from build123d import *

# Parameters (mm, degrees)
F0_R     = 1.475
F1_DEPTH = 10
F3_DEPTH = 3


with BuildPart() as f1:
    # F0 (on Front) → F1 (new body)
    with BuildSketch(Plane.XZ):
        Circle(F0_R)
    extrude(amount=F1_DEPTH)

    # F2 (on face) → F3 (cut)
    with BuildSketch(Plane(origin=(0, 0, 0), x_dir=(-1, 0, 0), z_dir=(0, 1, 0))):
        Polygon((-1.073836, 0.037674), (-0.569545, -0.911132), (0.504291, -0.948806), (1.073836, -0.037674), (0.569545, 0.911132), (-0.504291, 0.948806), align=None)
    extrude(amount=-F3_DEPTH, mode=Mode.SUBTRACT)


solid = f1.part
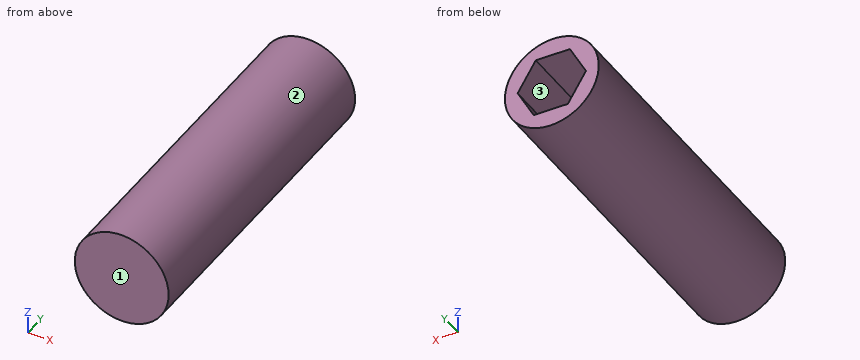
Can you work these out from the model? Positions are in its coordinate system, mm. Face numbers are marked on the shaded views. Give positions to 0.01 mm unless a question says otherwise; leave off trailing zeros. Loops run counter-clockwise (first coordinate to the right, second up) from the corner with the lowest first, then second, coordinate; pieces in that order, holes last. Notation, with made-up numbers: (60.25, 64) -> (88.25, 64) arc R14 ccw to (88.25, 85) -> close; hole circle Ø11 at (59.25, 19.25). An arc over 180 degrees is marked (long way). Use one line per item in the form item = value.
1) If we section it at C-C (y = -7.25): Please give me the cut outline in (x, z) (3 decimals).
Answers:
outline = circle Ø2.95 at (0, 0)
2) We'd pull the mould along X, two halves only. Please class the marked faces 1, 2 and 3: released by +X, released by -X, zero draft, split by the parting line, or undercut.
Answers:
face_1 = zero draft
face_2 = split by the parting line
face_3 = undercut
3) If we section it at B-B (z = 0.7): Please give me the cut outline in (x, y).
Answers:
outline = (-1.3, -10) -> (1.3, -10) -> (1.3, 0) -> (0.66, 0) -> (0.66, -3) -> (-0.68, -3) -> (-0.68, 0) -> (-1.3, 0) -> close
4) If we section it at A-A (x = 0.3): Please give me the cut outline in (y, z), plus the area to 3 significant figures.
Answers:
outline = (-10, -1.44) -> (0, -1.44) -> (0, -0.92) -> (-3, -0.92) -> (-3, 0.94) -> (0, 0.94) -> (0, 1.44) -> (-10, 1.44) -> close
area = 23.3 mm²
5) Will these pins go through, and if not, where does the flat tip stop? pin 1 (1.5 mm diameter, centred on x = 0, z = 0, fed in from +Y); pin 2 (1 mm diameter, centred on x = 0.5, y = -8, fed in from +Z) (3 decimals).
Answers:
pin_1 = -3
pin_2 = 1.475
6) I need wall thicknesses on line 1 along X through (y, z) = (-0.75, 0.75); line 2 along X through (y, z) = (-2, -0.15); line 3 along Y through (x, z) = (0.35, -0.65). Which ranges of each line are inside material? Lowest first, please.
Answers:
line_1 = -1.27 to -0.66, 0.63 to 1.27
line_2 = -1.47 to -1, 0.97 to 1.47
line_3 = -10 to -3
